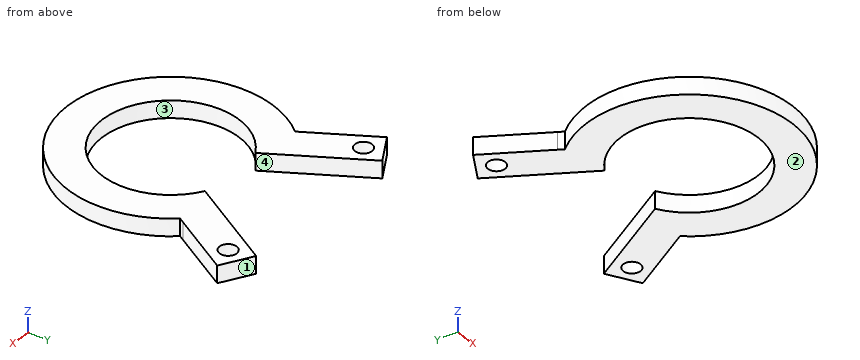
```python
from build123d import *

# Parameters (mm, degrees)
SKETCH2_R           = 19.05
SKETCH2_R_2         = 15.875
SKETCH2_R_3         = 12.7
BOSS_EXTRUDE1_DEPTH = 3.175
SKETCH3_R           = 1.5875
BOSS_EXTRUDE2_DEPTH = 3.175
CUT_EXTRUDE1_DEPTH  = 3.175


with BuildPart() as part:
    # Sketch2 → Boss-Extrude1 (new body)
    with BuildSketch(Plane.XY):
        Circle(SKETCH2_R)
        Circle(SKETCH2_R_2, mode=Mode.SUBTRACT)
        Circle(SKETCH2_R_2)
        Circle(SKETCH2_R_3, mode=Mode.SUBTRACT)
    extrude(amount=BOSS_EXTRUDE1_DEPTH)

    # Sketch3 → Boss-Extrude2 (add)
    with BuildSketch(Plane.XY.offset(3.175)):
        with BuildLine():
            ThreePointArc((-14.479517435, 12.379259867), (-12.17763419, 14.649495743), (-9.525, 16.497783942))
            Line((-9.525, 16.497783942), (-15.875, 27.49630657))
            Line((-15.875, 27.49630657), (-21.374261314, 24.32130657))
            Line((-21.374261314, 24.32130657), (-15.024261314, 13.322783942))
            Line((-15.024261314, 13.322783942), (-14.479517435, 12.379259867))
        make_face()
        with Locations((-17.037130657, 23.159175913)):
            Circle(SKETCH3_R, mode=Mode.SUBTRACT)
        with BuildLine():
            Line((15.875, 27.49630657), (9.525, 16.497783942))
            ThreePointArc((9.525, 16.497783942), (12.17763419, 14.649495743), (14.479517435, 12.379259867))
            Line((14.479517435, 12.379259867), (15.024261314, 13.322783942))
            Line((15.024261314, 13.322783942), (21.374261314, 24.32130657))
            Line((21.374261314, 24.32130657), (15.875, 27.49630657))
        make_face()
        with Locations((17.037130657, 23.159175913)):
            Circle(SKETCH3_R, mode=Mode.SUBTRACT)
    extrude(amount=-BOSS_EXTRUDE2_DEPTH)

    # Sketch5 → Cut-Extrude1 (cut)
    with BuildSketch(Plane.XY.offset(3.175)):
        with BuildLine():
            Line((-9.525, 16.497783942), (0, 0))
            Line((0, 0), (9.525, 16.497783942))
            ThreePointArc((9.525, 16.497783942), (0, 19.05), (-9.525, 16.497783942))
        make_face()
    extrude(amount=-CUT_EXTRUDE1_DEPTH, mode=Mode.SUBTRACT)


solid = part.part
```
Verification items for the finished model (mm, model axes). Face numbers are marked on the shaded views. Round coordinates to 2 decimals unless told otherwise and drop trailing zeros. Loops run counter-clockwise (first coordinate to the right, second up) from the corner with the lowest first, then second, coordinate; pieces in that order, holes last. Notation, with made-up numbers: (-35, -38.5) -> (-25, -38.5) arc R32 cw to (-25, -7.5) -> close; hole circle Ø4 at (74, -39.5). An arc over 180 degrees is marked (long way). Answer as a JSON object with one key per item and string values.
Q1. Scan lines: line 1 (X direction, y = 0, z = 2.45); line 2 (Y direction, x = -16, z = 2.35); line 3 (Y direction, x = -17.5, z = 1.1). Record each from-to range of solid material in increasing order. Write a range as from..to.
Data:
{"line 1": "x = -19.05..-12.7, 12.7..19.05", "line 2": "y = -10.34..10.34, 15.01..21.96, 24.36..27.42", "line 3": "y = -7.53..7.53, 17.61..21.64, 24.68..26.56"}
Q2. Draft check along X on the marked faces 1, 2, 3 and 4. Enter one of: pulls with the +X half, pulls with the -X half, needs draft (parallel to the pull), parting line crosses it, or undercut.
Data:
{"face 1": "pulls with the +X half", "face 2": "needs draft", "face 3": "undercut", "face 4": "undercut"}
Q3. Section check D-D (x = 0). Record the boundary of the cut face in (y, z) (3 decimals), then the cut area to 3 significant figures.
Data:
{"outline": "(-19.05, 0) -> (-12.7, 0) -> (-12.7, 3.175) -> (-19.05, 3.175) -> close", "area": "20.2 mm2"}
Q4. Section check B-B (x = 11.5). Record the boundary of the cut face in (y, z) (3 decimals), then the cut area to 3 significant figures.
Data:
{"outline": "(-15.187, 0) -> (-5.389, 0) -> (-5.389, 3.175) -> (-15.187, 3.175) -> close; (5.389, 0) -> (19.919, 0) -> (19.919, 3.175) -> (5.389, 3.175) -> close", "area": "77.2 mm2"}
Q5. Section check A-A (y = 0). Record the boundary of the cut face in (x, z) (3 decimals), then the cut area to 3 significant figures.
Data:
{"outline": "(-19.05, 0) -> (-12.7, 0) -> (-12.7, 3.175) -> (-19.05, 3.175) -> close; (12.7, 0) -> (19.05, 0) -> (19.05, 3.175) -> (12.7, 3.175) -> close", "area": "40.3 mm2"}
Q6. Section check C-C (z = 1.1). State how many separate pieces and enclosed holes the cut face has, then the cut area to 3 significant figures.
Data:
{"separate pieces": "1", "enclosed holes": "2", "area": "678 mm2"}
